CAD build for the part. Positions are in the model's coordinates, mm. Give positions to 0.01 mm unless a question says otherwise; leave off trailing zeros. Loops run counter-clockwise (first coordinate to the right, second up) from the corner with the lowest first, then second, coordinate; pieces in that order, holes last.
```python
from build123d import *

# Parameters (mm, degrees)
SKETCH1_R             = 1.6
SKETCH1_R_2           = 1.65
BOSS_EXTRUDE1_DEPTH   = 4.75
DEBURS_NO_SPRING_SIZE = 0.2


with BuildPart() as part:
    # Sketch1 → Boss-Extrude1 (new, symmetric)
    with BuildSketch(Plane.XY):
        with BuildLine():
            Line((-3.5, 0), (-3.5, -12))
            ThreePointArc((-3.5, -12), (0, -15.5), (3.5, -12))
            Line((3.5, -12), (3.5, 0))
            ThreePointArc((3.5, 0), (0, 3.5), (-3.5, 0))
        make_face()
        Circle(SKETCH1_R, mode=Mode.SUBTRACT)
        with Locations((0, -12)):
            Circle(SKETCH1_R_2, mode=Mode.SUBTRACT)
    extrude(amount=BOSS_EXTRUDE1_DEPTH, both=True)

    # Deburs no Spring
    deburs_no_spring_edges = [part.edges().sort_by_distance(p)[0] for p in [
        (-1.65, -12, -4.75),
        (-1.6, 0, -4.75),
        (-1.65, -12, 4.75),
        (-3.5, -6, 4.75),
        (0, -15.5, 4.75),
        (3.5, -6, 4.75),
        (0, 3.5, 4.75),
        (-1.6, 0, 4.75),
        (0, 3.5, -4.75),
        (3.5, -6, -4.75),
        (0, -15.5, -4.75),
        (-3.5, -6, -4.75),
    ]]
    chamfer(deburs_no_spring_edges, length=DEBURS_NO_SPRING_SIZE)


solid = part.part
```
1. Pull direction X, two halves, no side cores. Call faces 1 (the face through (3.5, -6, 0)), 2 (the face through (0.1, 3.5, 0.1)), 3 (the face through (-1.27, -0.97, -0.06)): released by +X, released by -X, zero draft, split by the parting line, or undercut.
Responses:
face 1: released by +X
face 2: split by the parting line
face 3: undercut
2. Saw through at C-C, the plane x = 1.25. Count the separate pieces of the cut face and the enclosed holes in it, and give its area (3 significant figures).
Responses:
separate pieces: 3
enclosed holes: 0
area: 136 mm2
3. Probe line 1 along Y through (x, z) = (0, -1.75); line 2 along Y through (x, z) = (1, 3); line 3 along X through (y, z) = (0.75, -2.75). List the from-to ranges inside material, lowest first.
Responses:
line 1: y = -15.5 to -13.65, -10.35 to -1.6, 1.6 to 3.5
line 2: y = -15.35 to -13.31, -10.69 to -1.25, 1.25 to 3.35
line 3: x = -3.42 to -1.41, 1.41 to 3.42
4. Saw through at A-A, the plane x = 0. List the corners of the cut face in (y, z).
Responses:
outline: (-15.5, -4.55) - (-15.3, -4.75) - (-13.85, -4.75) - (-13.65, -4.55) - (-13.65, 4.55) - (-13.85, 4.75) - (-15.3, 4.75) - (-15.5, 4.55) - close; (-10.35, -4.55) - (-10.15, -4.75) - (-1.8, -4.75) - (-1.6, -4.55) - (-1.6, 4.55) - (-1.8, 4.75) - (-10.15, 4.75) - (-10.35, 4.55) - close; (1.6, -4.55) - (1.8, -4.75) - (3.3, -4.75) - (3.5, -4.55) - (3.5, 4.55) - (3.3, 4.75) - (1.8, 4.75) - (1.6, 4.55) - close
5. Saw through at B-B, the plane z = -3.5. List the corners of the cut face in (x, y).
Responses:
outline: (-3.5, -12) arc R3.5 ccw to (3.5, -12) - (3.5, 0) arc R3.5 ccw to (-3.5, 0) - close; hole circle Ø3.3 at (0, -12); hole circle Ø3.2 at (0, 0)
